Here's how the part is built. I have some questions about the finished solid (model axes, mm). Give positions to 0.01 mm unless a question says otherwise; leave off trailing zeros. Write each loop counter-clockwise with the first axis right and the second up, starting at its lowest first coordinate (ties: lowest second). Pieces come first, ordered by that corner, then holes. Notation, with made-up numbers: (-20.5, -11.75) -> (38.5, -11.75) arc R24 ccw to (38.5, 23.25) -> close; hole circle Ø2 at (-21, -22.75). An arc over 180 degrees is marked (long way). Use one line per item in the form item = value.
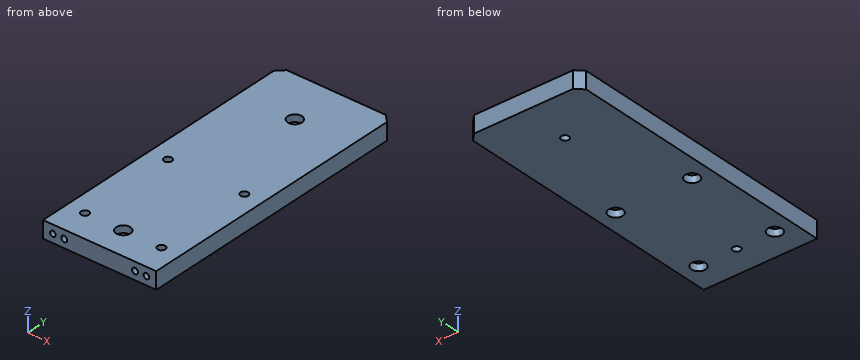
```python
from build123d import *

# Parameters (mm, degrees)
BOSS_EXTRUDE1_DEPTH                             = 12
CBORE_FOR_M5_SOCKET_HEAD_CAP_SCREW1_D           = 5.5
CBORE_FOR_M5_SOCKET_HEAD_CAP_SCREW1_CBORE_D     = 10
CBORE_FOR_M5_SOCKET_HEAD_CAP_SCREW1_CBORE_DEPTH = 5
M5X0_8_TAPPED_HOLE1_D                           = 4.2
M5X0_8_TAPPED_HOLE1_DEPTH                       = 14
M5X0_8_TAPPED_HOLE1_TIP                         = 1.2618073
SKETCH6_R                                       = 2
CUT_EXTRUDE1_DEPTH                              = 8
CBORE_FOR_M5_SOCKET_HEAD_CAP_SCREW2_D           = 5.5
CBORE_FOR_M5_SOCKET_HEAD_CAP_SCREW2_CBORE_D     = 10
CBORE_FOR_M5_SOCKET_HEAD_CAP_SCREW2_CBORE_DEPTH = 5


with BuildPart() as part:
    # Sketch1 → Boss-Extrude1 (new body)
    with BuildSketch(Plane.XY):
        Polygon((-40, 0), (40, 0), (40, 195), (35, 200), (-35, 200), (-40, 195), align=None)
    extrude(amount=BOSS_EXTRUDE1_DEPTH)

    # CBORE for M5 Socket Head Cap Screw1 (through all)
    with Locations(Plane.XY.offset(12)):
        with Locations((0, 20), (0, 165)):
            CounterBoreHole(CBORE_FOR_M5_SOCKET_HEAD_CAP_SCREW1_D / 2, CBORE_FOR_M5_SOCKET_HEAD_CAP_SCREW1_CBORE_D / 2, CBORE_FOR_M5_SOCKET_HEAD_CAP_SCREW1_CBORE_DEPTH)

    # M5x0.8 Tapped Hole1
    with Locations(Plane.XZ):
        with Locations((-25, 6), (25, 6)):
            Hole(M5X0_8_TAPPED_HOLE1_D / 2, depth=M5X0_8_TAPPED_HOLE1_DEPTH)
            with Locations((0, 0, -(M5X0_8_TAPPED_HOLE1_DEPTH + M5X0_8_TAPPED_HOLE1_TIP / 2))):  # 118° drill point
                Cone(0, M5X0_8_TAPPED_HOLE1_D / 2, M5X0_8_TAPPED_HOLE1_TIP, mode=Mode.SUBTRACT)

    # Sketch6 → Cut-Extrude1 (cut)
    with BuildSketch(Plane(origin=(0, 0, 0), x_dir=(1, 0, 0), z_dir=(0, 1, 0))):
        with Locations((33, -6)):
            Circle(SKETCH6_R)
        with Locations((-33, -6)):
            Circle(SKETCH6_R)
    extrude(amount=CUT_EXTRUDE1_DEPTH, mode=Mode.SUBTRACT)

    # CBORE for M5 Socket Head Cap Screw2 (through all)
    with Locations(Plane(origin=(0, 0, 0), x_dir=(-1, 0, 0), z_dir=(0, 0, -1))):
        with Locations((27, 20), (27, 90), (-27, 90), (-27, 20)):
            CounterBoreHole(CBORE_FOR_M5_SOCKET_HEAD_CAP_SCREW2_D / 2, CBORE_FOR_M5_SOCKET_HEAD_CAP_SCREW2_CBORE_D / 2, CBORE_FOR_M5_SOCKET_HEAD_CAP_SCREW2_CBORE_DEPTH)


solid = part.part
```
Q1. I want a section at B-B, the plane x = 0. Write out the boundary of the cut face in (y, z).
Result set:
outline = (0, 0) -> (17.25, 0) -> (17.25, 7) -> (15, 7) -> (15, 12) -> (0, 12) -> close; (22.75, 0) -> (162.25, 0) -> (162.25, 7) -> (160, 7) -> (160, 12) -> (25, 12) -> (25, 7) -> (22.75, 7) -> close; (167.75, 0) -> (200, 0) -> (200, 12) -> (170, 12) -> (170, 7) -> (167.75, 7) -> close
Q2. I want a section at C-C, the plane y = 90. Write out the boundary of the cut face in (x, z).
Result set:
outline = (-40, 0) -> (-32, 0) -> (-32, 5) -> (-29.75, 5) -> (-29.75, 12) -> (-40, 12) -> close; (-24.25, 5) -> (-22, 5) -> (-22, 0) -> (22, 0) -> (22, 5) -> (24.25, 5) -> (24.25, 12) -> (-24.25, 12) -> close; (29.75, 5) -> (32, 5) -> (32, 0) -> (40, 0) -> (40, 12) -> (29.75, 12) -> close
Q3. Will these pins go through, and if not, where does the flat tip stop? pin 1 Ø5 at (x, y) = (0, 165) entering from -Z; pin 2 Ø9 at (x, y) = (0, 20) entering from +Z; pin 3 Ø3 at (x, y) = (25, 90) entering from -Z; pin 4 Ø3 at (x, z) = (33, 6) entering from -Y.
Result set:
pin_1 = through
pin_2 = 7
pin_3 = 5
pin_4 = 8
Q4. If I drill on line 1 along X through (y, z) = (5, 6); line 2 along Y through (x, z) = (-27, 2.9); line 3 along Z through (x, y) = (33, 6), over which ranges is the centre line in solid material (lowest first)? Write a range as from..to.
Result set:
line_1 = -40..-35, -31..-27.1, -22.9..22.9, 27.1..31, 35..40
line_2 = 0..15, 25..85, 95..200
line_3 = 0..4, 8..12
Q5. I want a section at A-A, the plane y = 165. Write out the boundary of the cut face in (x, z).
Result set:
outline = (-40, 0) -> (-2.75, 0) -> (-2.75, 7) -> (-5, 7) -> (-5, 12) -> (-40, 12) -> close; (2.75, 0) -> (40, 0) -> (40, 12) -> (5, 12) -> (5, 7) -> (2.75, 7) -> close
